Model file for the job. Use its own axes, mm. Face numbers are marked on the shaded views. Round coordinates to 2 decimals unless told otherwise and drop trailing zeros. Order: outer loops, then holes, each group sorted by start corner. A loop starts at its lowest first (then second) coordinate and runs counter-clockwise, first axis right, second up. Notation, with made-up numbers: (-22.75, 87) -> (-15.75, 87) arc R25 cw to (-15.75, 110) -> close; hole circle Ø5 at (-8.75, 79.5). An arc over 180 degrees is marked (long way). Put each result on its own line as item: value. Start each with the question number.
Q1. Pull direction Z, two halves, no side cores. Call the marked faces 1, 2 and 3: released by +Z, released by -Z, zero draft, split by the parting line, or undercut.
Q2. Cut at C-C, the plane x = 92. List the corners of the cut face in (y, z).
Q3. Cut at A-A, the plane y = 0. List the corners of the cut face in (x, z).
Q4. Flat gauge pins, fed straight in: P1, Ø8, axis at y = 0, z = 0, coming from the +X side; P2, Ø10, axis at x = 59.5, y = 6, coming from the -Z side; P3, Ø2, axis at x = 49.5, z = -2.5, coming from the -Y side. Where does each tip first touch, or does it go through?
Q5. Cut at D-D, the plane z = -7.75. List the corners of the cut face in (x, y).
Q6. Probe L1, parallel to X at y = 6, z = -9.75; L2, parallel to Y at x = 36, z = -2.75; L3, parallel to Z at x = 57, y = -1.5. List the from-to ranges inside material, lowest first.
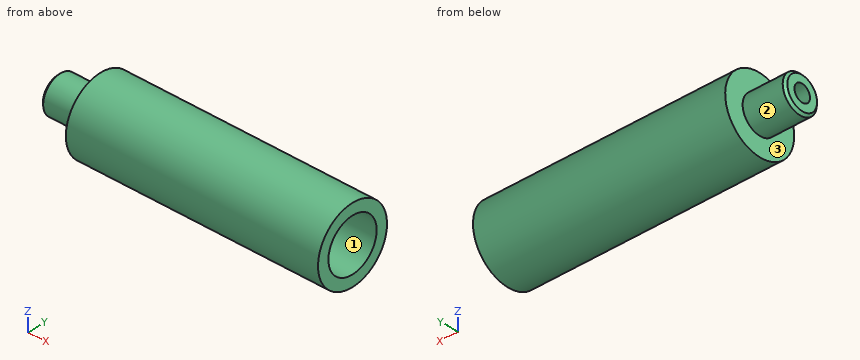
from build123d import *


# Read off the part's stored shape, not the designer's step: G1/4 Straight Pipe Tapped Thread Stud2
with BuildPart() as part:
    # Sketch1 → Revolve1 (revolve)
    with BuildSketch(Plane.XY, mode=Mode.PRIVATE) as revolve1_sk:
        Polygon((15, -13.3), (104, -13.3), (104, -9.3), (19, -9.3), (19, -3), (0, -3), (0, -7), (15, -7), align=None)
    revolve(revolve1_sk.sketch.rotate(Axis((0, 0, 0), (1, 0, 0)), 270), axis=Axis((0, 0, 0), (1, 0, 0)))

    # G1/4 Straight Pipe Tapped Thread Stud2 o → G1/4 Straight Pipe Tapped Thread Stud2 (revolve, cut)
    with BuildSketch(Plane.YX):
        Polygon((5.7225, 0), (7, 0), (7, 15), (6.5785, 15), (6.5785, 0.856), align=None)
    revolve(axis=Axis((0, 0, 0), (1, 0, 0)), mode=Mode.SUBTRACT)


solid = part.part
Ans:
1. face 1: undercut
1. face 2: split by the parting line
1. face 3: zero draft
2. outline: circle Ø26.6 at (0, 0); hole circle Ø18.6 at (0, 0)
3. outline: (0, -5.72) -> (0.86, -6.58) -> (15, -6.58) -> (15, -13.3) -> (104, -13.3) -> (104, -9.3) -> (19, -9.3) -> (19, -3) -> (0, -3) -> close; (0, 3) -> (19, 3) -> (19, 9.3) -> (104, 9.3) -> (104, 13.3) -> (15, 13.3) -> (15, 6.58) -> (0.86, 6.58) -> (0, 5.72) -> close
4. P1: stops at x = 19
4. P2: stops at z = -13.26
4. P3: stops at y = -13.22
5. outline: (15, -10.81) -> (104, -10.81) -> (104, -5.14) -> (19, -5.14) -> (19, 5.14) -> (104, 5.14) -> (104, 10.81) -> (15, 10.81) -> close
6. L1: x = 15 to 104
6. L2: y = -13.01 to -8.88, 8.88 to 13.01
6. L3: z = -13.22 to -9.18, 9.18 to 13.22
